Input: part model. Units: mm. Frame: model coordinates. Round coordinates to 2 decimals unless told otherwise and drop trailing zeros. Loops run counter-clockwise (first coordinate to the right, second up) from the corner with the lowest first, then second, coordinate; pieces in that order, holes last. Notation, with made-up numbers: (35.5, -3.75) - (63.5, -3.75) arc R23 cw to (63.5, 19.25) - close; hole circle Ø1 at (2, -1.5). An arc over 180 degrees is marked (long way). Use CSV: the item, a comma, the result in double quotes. Start each with the question number.
1. Cut plane C-C (y = -177). Return loops of the section in (x, z).
2. Pin query (flat end, axial travel): P1, Ø0.9, axis at x = 0, z = 0, coming from the -Y side. Return the tip coordinate at first contact, or that it passes through.
3. Cut plane B-B (z = 0). Return loops of the section in (x, y), and give its area (3 significant figures).
4. Material intervals for probe 1 along Z at (x, y) = (-0.2, -370); probe 2 along X at (y, z) = (-285, -0.15); probe 3 along Z at (x, y) = (0, -143), sorted ascending. Write a range as from..to.
5. Cut plane A-A (x = 0). Return loops of the section in (y, z), and give its area (3 significant figures).
```python
from build123d import *

# Parameters (mm, degrees)
F0_R     = 1.27
F0_R_2   = 0.762
F1_DEPTH = 508
F2_SIZE  = 0.254
F3_R     = 0.0508


with BuildPart() as f1:
    # F0 (on Front) → F1 (new body)
    with BuildSketch(Plane.XZ):
        Circle(F0_R)
        Circle(F0_R_2, mode=Mode.SUBTRACT)
    extrude(amount=F1_DEPTH)

    # F2
    f2_edges = [f1.edges().sort_by_distance(p)[0] for p in [
        (-0.762, 0, 0),
    ]]
    chamfer(f2_edges, length=F2_SIZE)

    # F3
    f3_edges = [f1.edges().sort_by_distance(p)[0] for p in [
        (-1.27, 0, 0),
    ]]
    fillet(f3_edges, radius=F3_R)


solid = f1.part
```
Established:
1,outline,"circle Ø2.54 at (0, 0); hole circle Ø1.52 at (0, 0)"
2,P1,"passes through"
3,outline,"(-1.27, -508) - (-0.76, -508) - (-0.76, -0.25) - (-1.02, 0) - (-1.22, 0) arc R0.05 ccw to (-1.27, -0.05) - close; (0.76, -508) - (1.27, -508) - (1.27, -0.05) arc R0.05 ccw to (1.22, 0) - (1.02, 0) - (0.76, -0.25) - close"
3,area,"516 mm2"
4,probe 1,"z = -1.25..-0.74, 0.74..1.25"
4,probe 2,"x = -1.26..-0.75, 0.75..1.26"
4,probe 3,"z = -1.27..-0.76, 0.76..1.27"
5,outline,"(-508, -1.27) - (-0.05, -1.27) arc R0.05 ccw to (0, -1.22) - (0, -1.02) - (-0.25, -0.76) - (-508, -0.76) - close; (-508, 0.76) - (-0.25, 0.76) - (0, 1.02) - (0, 1.22) arc R0.05 ccw to (-0.05, 1.27) - (-508, 1.27) - close"
5,area,"516 mm2"
